Study the drawing (mm; zero at the part's minimum x, y, z) and answer. A direction names the side the tool comes from. Coordinates: 2 decimals unless noted, no trailing zeros. Order: outer loops, then holes, each group sorted by start corner. A loop starts at its lowest first (then second) coordinate and runs counter-clockwise, first axis right, second up.
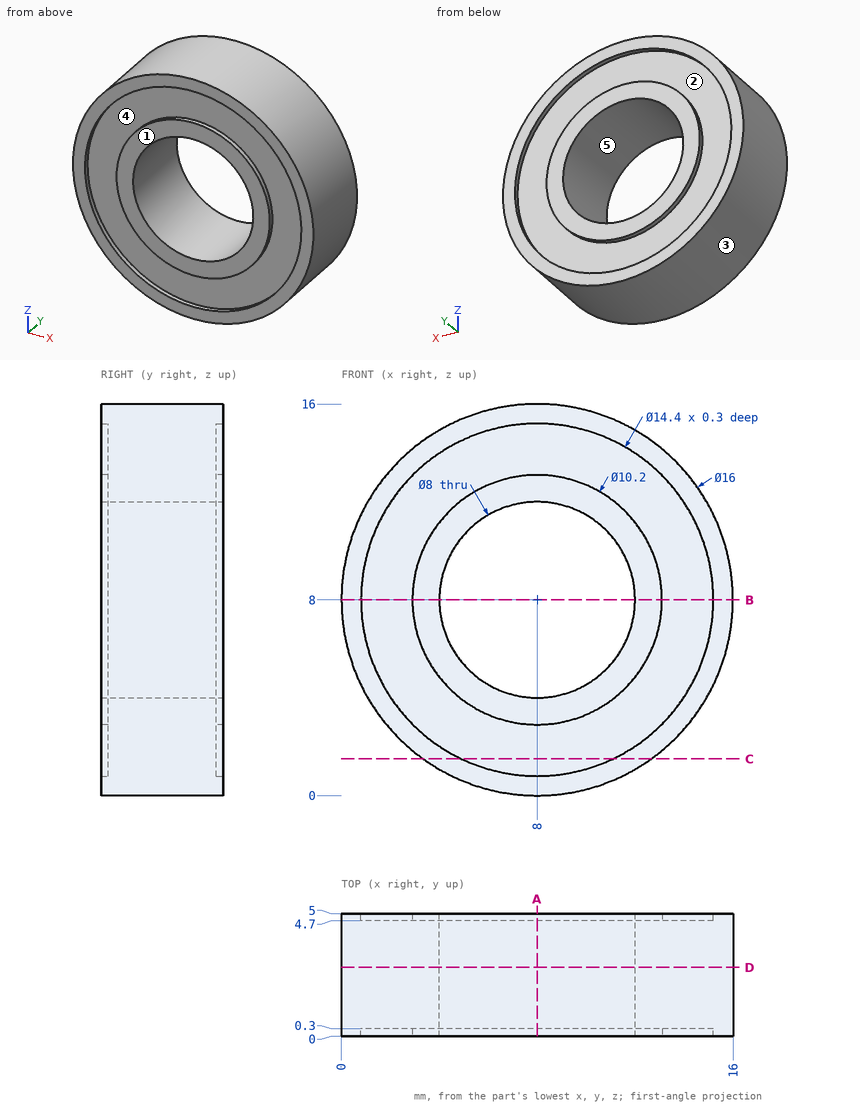
1) Flat-ended cylindrical pins translate along their axes: pin 1 Ø4.5 at (x, z) = (9.5, 5) entering from -Y; pin 2 Ø1.5 at (y, z) = (3.5, 4) entering from -X. Find the tip coordinate at first contact, or state that the pin passes through.
A:
pin 1: stops at y = 0
pin 2: stops at x = 0.69
2) Determine the mould class of the marked faces 1, 2 and 3 for opening direction X: pulls with the +X half, pulls with the -X half, needs draft (parallel to the pull), parting line crosses it, or undercut.
A:
face 1: needs draft
face 2: undercut
face 3: parting line crosses it
3) A cutting plane is placed at C-C, the plane z = 1.5. Determine the outline of the cut face in (x, y).
A:
outline: (3.34, 0) - (4.9, 0) - (4.9, 0.3) - (11.1, 0.3) - (11.1, 0) - (12.66, 0) - (12.66, 5) - (11.1, 5) - (11.1, 4.7) - (4.9, 4.7) - (4.9, 5) - (3.34, 5) - close
4) A cutting plane is placed at B-B, the plane z = 8. Determine the outline of the cut face in (x, y), and give its area (3 significant figures).
A:
outline: (0, 0) - (0.8, 0) - (0.8, 0.3) - (2.9, 0.3) - (2.9, 0) - (4, 0) - (4, 5) - (2.9, 5) - (2.9, 4.7) - (0.8, 4.7) - (0.8, 5) - (0, 5) - close; (12, 0) - (13.1, 0) - (13.1, 0.3) - (15.2, 0.3) - (15.2, 0) - (16, 0) - (16, 5) - (15.2, 5) - (15.2, 4.7) - (13.1, 4.7) - (13.1, 5) - (12, 5) - close
area: 37.5 mm2
5) Straight lines are drawn through the part: line 1 (X direction, y = 0.25, z = 8); line 2 (X direction, y = 1.35, z = 8); line 3 (Y direction, x = 2, z = 8.25). For each, find the intervals that lie inside material, in ascending order.
A:
line 1: x = 0 to 0.8, 2.9 to 4, 12 to 13.1, 15.2 to 16
line 2: x = 0 to 4, 12 to 16
line 3: y = 0.3 to 4.7
6) Which of the six approach directions +Z, -Z, +X, -X, +Y, -Y give full straight-line access (tool end or side, diameter ignored) to the marked faces 4 and 5?
A:
face 4: -Y
face 5: +Y, -Y
7) A cutting plane is placed at D-D, the plane y = 2.8. Determine the outline of the cut face in (x, z).
A:
outline: circle Ø16 at (8, 8); hole circle Ø8 at (8, 8)
8) A cutting plane is placed at A-A, the plane x = 8. Determine the outline of the cut face in (y, z), and give its area (3 significant figures).
A:
outline: (0, 0) - (5, 0) - (5, 0.8) - (4.7, 0.8) - (4.7, 2.9) - (5, 2.9) - (5, 4) - (0, 4) - (0, 2.9) - (0.3, 2.9) - (0.3, 0.8) - (0, 0.8) - close; (0, 12) - (5, 12) - (5, 13.1) - (4.7, 13.1) - (4.7, 15.2) - (5, 15.2) - (5, 16) - (0, 16) - (0, 15.2) - (0.3, 15.2) - (0.3, 13.1) - (0, 13.1) - close
area: 37.5 mm2
